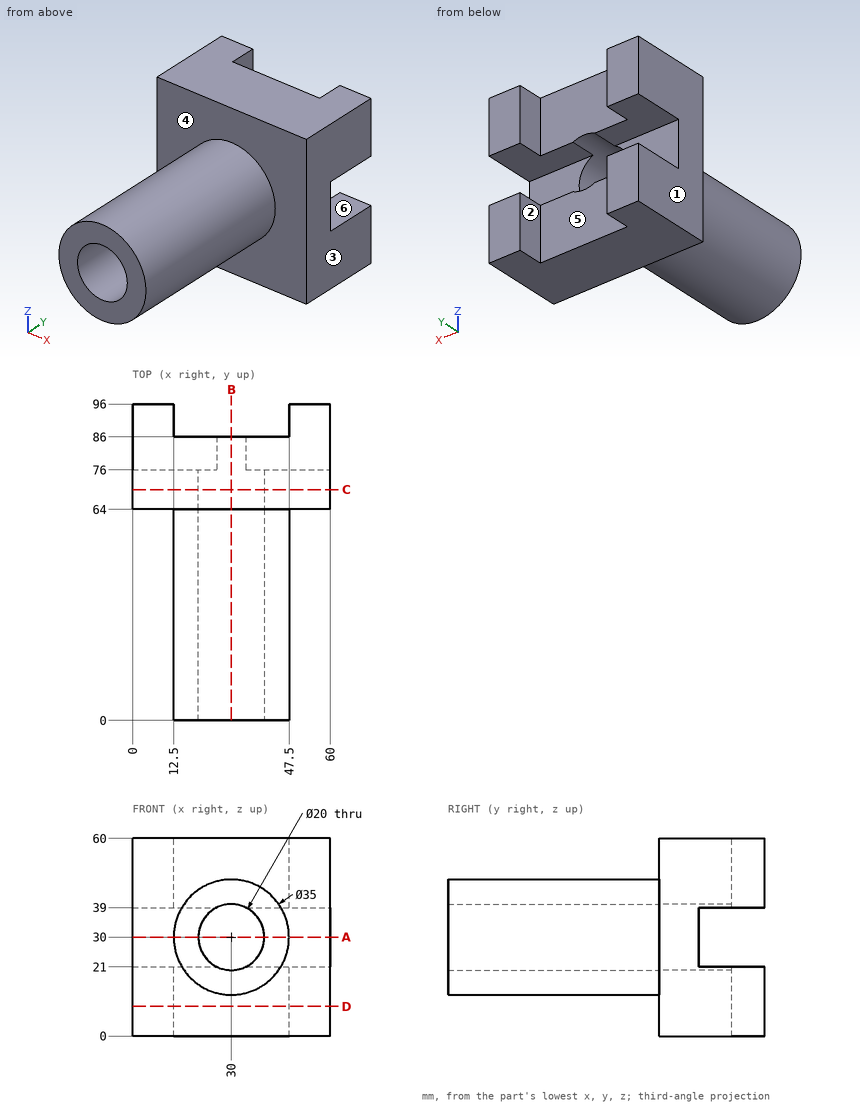
Check sheet for the drawn part. Datum: minimum x, y, z corner. Units: mm. A direction names the side the tool comes from. Give positions to 0.01 mm unless a question says otherwise; leave off trailing zeros. Write each loop counter-clockwise with the first axis right and the second up, starting at its lowest first coordinate (ties: lowest second). Pieces come first, ordered by that corner, then holes.
(1) Access from +Z, -Z, +X, -X, +Y, -Y to the whole of each face (thin tool, end or side, straight path). Record for the marked faces 4, 5 and 6.
(2) Cross-section at D-D (z = 9). Enter the section's corners in (x, y).
(3) Cross-section at C-C (y = 70). Enter the section's corners in (x, z).
(4) Gauge pin test, flat ends, axial feed: pin 1 (10 mm diameter, centred on x = 29.5, y = 48, fed in from +Z); pin 2 (14.5 mm diameter, centred on x = 11, z = 26.5, fed in from +Y); pin 3 (4 mm diameter, centred on y = 13.5, z = 36.5, fed in from -X); pin 4 (6.5 mm diameter, centred on x = 23.5, z = 8.5, fed in from +Y). Record the tip position at first contact, or that the pin passes through.
(5) Material ranges on line 1 (Z direction, x = 30, y = 79.75); line 2 (Z direction, x = 34.5, y = 84); line 3 (Y direction, x = 56, z = 16), recorded low to high.
(6) Mould release check, pull along X, two halves, no side actions. Record for the marked faces 1, 2 and 3: +X half, -X half, draft (parallel to the pull), parting line (faces both ways), or undercut.
(7) Cross-section at A-A (z = 30). Enter the section's corners in (x, y).
(8) Cross-section at B-B (x = 30). Enter the section's corners in (y, z), plus the area to 3 significant figures.
Worked out:
1. face 4: -Y
1. face 5: +Z, -Z, +Y
1. face 6: +X, -X, +Y
2. outline: (0, 64) - (60, 64) - (60, 96) - (47.5, 96) - (47.5, 86) - (12.5, 86) - (12.5, 96) - (0, 96) - close
3. outline: (0, 0) - (60, 0) - (60, 60) - (0, 60) - close; hole circle Ø20 at (30, 30)
4. pin 1: stops at z = 47.5
4. pin 2: stops at y = 96
4. pin 3: stops at x = 13.09
4. pin 4: stops at y = 86
5. line 1: z = 0 to 20, 40 to 60
5. line 2: z = 0 to 21, 39 to 60
5. line 3: y = 64 to 96
6. face 1: -X half
6. face 2: undercut
6. face 3: +X half
7. outline: (0, 64) - (12.5, 64) - (12.5, 0) - (20, 0) - (20, 76) - (0, 76) - close; (40, 0) - (47.5, 0) - (47.5, 64) - (60, 64) - (60, 76) - (40, 76) - close
8. outline: (0, 12.5) - (64, 12.5) - (64, 0) - (86, 0) - (86, 20) - (0, 20) - close; (0, 40) - (86, 40) - (86, 60) - (64, 60) - (64, 47.5) - (0, 47.5) - close
8. area: 1,840 mm2
